from build123d import *

# Parameters (mm, degrees)
SKETCH1_W           = 57
SKETCH1_H           = 110
BOSS_EXTRUDE1_DEPTH = 4
SKETCH2_W           = 4
SKETCH2_H           = 110
BOSS_EXTRUDE2_DEPTH = 96
SKETCH3_R           = 3.41
BOSS_EXTRUDE3_DEPTH = 4
CUT_EXTRUDE1_REACH  = 121.785
SKETCH4_R           = 4
CUT_EXTRUDE2_REACH  = 126.459
SKETCH5_W           = 88
SKETCH5_H           = 88
BOSS_EXTRUDE4_DEPTH = 55
BOSS_EXTRUDE5_DEPTH = 100


with BuildPart() as part:
    # Sketch1 → Boss-Extrude1 (new body)
    with BuildSketch(Plane(origin=(0, 0, 0), x_dir=(1, 0, 0), z_dir=(0, 1, 0))):
        with Locations((-7.88, 0)):
            Rectangle(SKETCH1_W, SKETCH1_H)
    extrude(amount=BOSS_EXTRUDE1_DEPTH)

    # Sketch2 → Boss-Extrude2 (add)
    with BuildSketch(Plane.XZ):
        with Locations((18.62, 0)):
            Rectangle(SKETCH2_W, SKETCH2_H)
    extrude(amount=BOSS_EXTRUDE2_DEPTH)

    # Sketch3 → Boss-Extrude3 (add)
    # profile 1 of 2: a face of its own
    with BuildSketch(Plane(origin=(-32.38, 0, 0), x_dir=(0, 0, -1), z_dir=(1, 0, 0))):
        with BuildLine():
            Line((45, 0), (45, -5))
            ThreePointArc((45, -5), (40, -10), (35, -5))
            Line((35, -5), (35, 0))
            Line((35, 0), (45, 0))
        make_face()
        with Locations((40, -5)):
            Circle(SKETCH3_R, mode=Mode.SUBTRACT)
    # profile 2 of 2: a face of its own
    with BuildSketch(Plane(origin=(-32.38, 0, 0), x_dir=(0, 0, -1), z_dir=(1, 0, 0))):
        with BuildLine():
            Line((-35, 0), (-35, -5))
            ThreePointArc((-35, -5), (-40, -10), (-45, -5))
            Line((-45, -5), (-45, 0))
            Line((-45, 0), (-35, 0))
        make_face()
        with Locations(Location((-40, -5, 0), (0, 0, 180))):
            Circle(SKETCH3_R, mode=Mode.SUBTRACT)
    extrude(amount=BOSS_EXTRUDE3_DEPTH)

    # Sketch4 → Cut-Extrude1 (cut, up to next)
    with BuildSketch(Plane(origin=(0, 4, 0), x_dir=(1, 0, 0), z_dir=(0, 1, 0)), mode=Mode.PRIVATE) as cut_extrude1_sk1:
        with Locations(Location((5.12, 0.25, 0), (0, 0, 270))):
            Circle(SKETCH4_R)
    cut_extrude1_tool1 = extrude(cut_extrude1_sk1.sketch, amount=-CUT_EXTRUDE1_REACH, mode=Mode.PRIVATE) & part.part
    add(cut_extrude1_tool1.solids().sort_by_distance((5.12, 4, -0.25))[0], mode=Mode.SUBTRACT)

    # Sketch5 → Cut-Extrude2 (cut, up to next)
    with BuildSketch(Plane(origin=(20.62, 0, 0), x_dir=(0, 0, -1), z_dir=(1, 0, 0)), mode=Mode.PRIVATE) as cut_extrude2_sk1:
        with Locations((0, -52)):
            Rectangle(SKETCH5_W, SKETCH5_H)
    cut_extrude2_tool1 = extrude(cut_extrude2_sk1.sketch, amount=-CUT_EXTRUDE2_REACH, mode=Mode.PRIVATE) & part.part
    add(cut_extrude2_tool1.solids().sort_by_distance((20.62, -52, 0))[0], mode=Mode.SUBTRACT)

    # Sketch6 → Boss-Extrude4 (add, symmetric)
    with BuildSketch(Plane.XY):
        Polygon((20.62, 2), (20.62, 4), (23.62, 4), (23.62, 0), (22.12, 0), (22.12, 2), align=None)
    extrude(amount=BOSS_EXTRUDE4_DEPTH, both=True)

    # Sketch7 → Boss-Extrude5 (add)
    with BuildSketch(Plane(origin=(0, 4, 0), x_dir=(1, 0, 0), z_dir=(0, 1, 0))):
        Polygon((23.62, 55), (20.62, 55), (20.62, 53), (22.12, 53), (22.12, 51), (23.62, 51), align=None)
        Polygon((23.62, -51), (23.62, -55), (20.62, -55), (20.62, -53), (22.12, -53), (22.12, -51), align=None)
    extrude(amount=-BOSS_EXTRUDE5_DEPTH)


solid = part.part
Verification items for the finished model (mm, model axes). A direction names the side the tool comes from. Round coordinates to 2 decimals unless told otherwise and drop trailing zeros. Loops run counter-clockwise (first coordinate to the right, second up) from the corner with the lowest first, then second, coordinate; pieces in that order, holes last. Notation, with made-up numbers: (76, 19.5) - (83, 19.5) arc R20 ccw to (83, 26.5) - close; hole circle Ø7 at (59, 42). An arc over 180 degrees is marked (long way). Use one line per item in the form item = value.
1. Section check D-D on z = -20.5. Record the cut outline in (x, y), and give its area (3 significant figures).
A:
outline = (-36.38, 0) - (16.62, 0) - (16.62, -8) - (20.62, -8) - (20.62, 2) - (22.12, 2) - (22.12, 0) - (23.62, 0) - (23.62, 4) - (-36.38, 4) - close
area = 269 mm²
2. Scan lines: probe 1 along Y at (x, z) = (-31.2, 40); probe 2 along Y at (x, z) = (-25.5, 12); probe 3 along Z at (x, y) = (19, -52). Record each from-to range of solid material in increasing order.
A:
probe_1 = -10 to -8.41, -1.59 to 4
probe_2 = 0 to 4
probe_3 = -55 to -44, 44 to 55
3. Section check C-C on y = -18. Record the cut outline in (x, z).
A:
outline = (16.62, -55) - (23.62, -55) - (23.62, -51) - (22.12, -51) - (22.12, -53) - (20.62, -53) - (20.62, -44) - (16.62, -44) - close; (16.62, 44) - (20.62, 44) - (20.62, 53) - (22.12, 53) - (22.12, 51) - (23.62, 51) - (23.62, 55) - (16.62, 55) - close
4. Section check B-B on z = -40. Record the cut outline in (x, y).
A:
outline = (-36.38, 0) - (-32.38, 0) - (-32.38, -1.59) - (-28.38, -1.59) - (-28.38, 0) - (16.62, 0) - (16.62, -8) - (20.62, -8) - (20.62, 2) - (22.12, 2) - (22.12, 0) - (23.62, 0) - (23.62, 4) - (-36.38, 4) - close; (-32.38, -10) - (-28.38, -10) - (-28.38, -8.41) - (-32.38, -8.41) - close
5. Draft check along X on faces 5 (the cylindrical face through (1.215, 2.028, -1.117)), 6 (the flat face through (-32.38, -1.6, 38.8)), 7 (the cylindrical face through (-30, -10, -40)). Enter one of: pulls with the +X half, pulls with the -X half, needs draft (parallel to the pull), parting line crosses it, or undercut.
A:
face_5 = undercut
face_6 = pulls with the -X half
face_7 = needs draft
6. Section check A-A on x = 5.12. Record the cut outline in (y, z), and give its area (3 significant figures).
A:
outline = (0, -55) - (4, -55) - (4, -4.25) - (0, -4.25) - close; (0, 3.75) - (4, 3.75) - (4, 55) - (0, 55) - close
area = 408 mm²
7. Gauge pin test, flat ends, axial feed: pin 1 Ø8 at (y, z) = (-5, -40) entering from -X; pin 2 Ø1.2 at (x, z) = (21, -22.5) entering from -Y; pin 3 Ø16 at (x, z) = (-2.5, 18) entering from -Y. Record the tip position at first contact, or that the pin passes through.
A:
pin_1 = -32.38
pin_2 = -8
pin_3 = 0
8. Access from +Z, -Z, +X, -X, +Y, -Y to the whole of each face (thin tool, end or side, straight path). Record for faces 1 (the flat face through (19, -53, 44)), 2 (the flat face through (-30, -3, 45)), 3 (the flat face through (20.62, -7, 0)), 4 (the cylindrical face through (-30.408, -5.15, 36.593)).
A:
face_1 = +X, -X, -Y
face_2 = +Z, -X, -Y
face_3 = -Y
face_4 = -X
